from build123d import *

# Parameters (mm, degrees)
F0_W     = 24.9174
F0_H     = 22.5044
F1_DEPTH = 24.9936
F2_R     = 4.1529
F3_DEPTH = 24.9946


with BuildPart() as f1:
    # F0 (on Right) → F1 (new body)
    with BuildSketch(Plane.YZ):
        with Locations((12.4587, 11.2522)):
            Rectangle(F0_W, F0_H)
        with BuildLine():
            ThreePointArc((24.9174, 22.5044), (12.4587, 34.9631), (0, 22.5044))
            Line((0, 22.5044), (24.9174, 22.5044))
        make_face()
    extrude(amount=-F1_DEPTH)

    # F2 (on face) → F3 (cut, through all)
    with BuildSketch(Plane.YZ):
        with Locations((12.4587, 22.5044)):
            Circle(F2_R)
    extrude(amount=-F3_DEPTH, mode=Mode.SUBTRACT)


solid = f1.part
CAD build for the part. Positions are in the model's coordinates, mm. Round coordinates to 2 decimals unless told otherwise and drop trailing zeros. Loops run counter-clockwise (first coordinate to the right, second up) from the corner with the lowest first, then second, coordinate; pieces in that order, holes last.
(1) Wall check: line 1 along Z through (x, y) = (-9, 12.5); line 2 along Y through (x, z) = (-17.75, 22.5); line 3 along Y through (x, z) = (-8, 24). Give the ranges that are in metal, low to high.
(2) Cut at C-C (z = 20). Give the cut face in (x, y), plus the area to 3 significant figures.
(3) Cut at B-B (y = 13.75). Give the cut face in (x, z).
(4) Cut at D-D (y = 22.5). Give the cut face in (x, z).
(5) Cut at A-A (x = -16.5). Give the cut face in (y, z), plus the area to 3 significant figures.
(6) Drop flat-ended pins along their axis: pin 1 (1 mm diameter, centred on x = -11.5, y = 5.5, fed in from +Z); pin 2 (1 mm diameter, centred on x = -13.5, y = 11.5, fed in from +Z); pin 3 (1.5 mm diameter, centred on x = -6.5, y = 18.5, fed in from +Z). Give the stop position or say it passes through.
Findings below:
1. line 1: z = 0 to 18.35, 26.66 to 34.96
1. line 2: y = 0 to 8.31, 16.61 to 24.92
1. line 3: y = 0.09 to 8.58, 16.33 to 24.83
2. outline: (-24.99, 0) - (0, 0) - (0, 9.15) - (-24.99, 9.15) - close; (-24.99, 15.77) - (0, 15.77) - (0, 24.92) - (-24.99, 24.92) - close
2. area: 457 mm2
3. outline: (-24.99, 0) - (0, 0) - (0, 18.56) - (-24.99, 18.56) - close; (-24.99, 26.45) - (0, 26.45) - (0, 34.9) - (-24.99, 34.9) - close
4. outline: (-24.99, 0) - (0, 0) - (0, 29.88) - (-24.99, 29.88) - close
5. outline: (0, 0) - (24.92, 0) - (24.92, 22.5) arc R12.46 ccw to (0, 22.5) - close; hole circle Ø8.31 at (12.46, 22.5)
5. area: 750 mm2
6. pin 1: stops at z = 33.16
6. pin 2: stops at z = 34.95
6. pin 3: stops at z = 33.78
